Verification items for the finished model (mm, model axes). Face numbers are marked on the shaded views. Coordinates: 2 decimals unless noted, no trailing zeros. Order: outer loops, then holes, each group sorted by start corner. A loop starts at its lowest first (then second) coordinate and runs counter-clockwise, first axis right, second up. Notation, with made-up numbers: M -32.5,32.25 L 17.5,32.25 A31 ccw 17.5,64.25 Z; hole C 58.25,20.5 d4. An arc over 180 degrees is marked long. Write item = value, one per line.
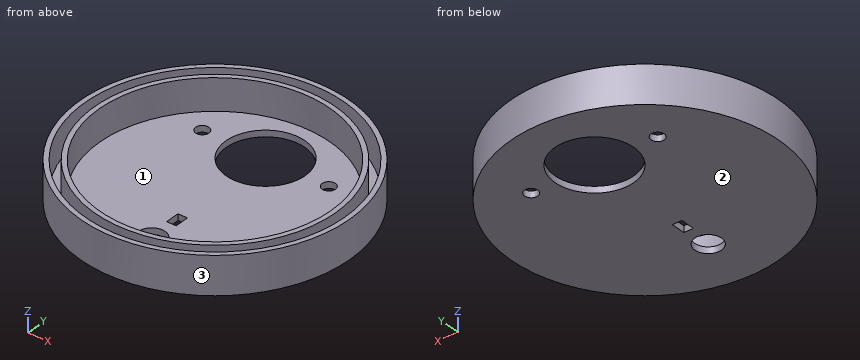
Autodesk Inventor part; units mm, degrees
sketch "Sketch1" plane through (0, 0, 0) normal (0, 0, 1) x (1, 0, 0)
  line L0 (0, 2.8582) -> (0, -2.8582) construction
  line L1 (-5.7775, 0) -> (5.7775, 0) construction
  circle A0 centre (0, 0) radius 42.5
  dimension "d0" = 85
extrude "Extrusion1" add sketch "Sketch1" along normal blind 2
sketch "Sketch2" plane through (0, 0, 2) normal (0, 0, 1) x (1, 0, 0)
  circle A0 centre (0, 0) radius 41
  circle A1 centre (0, 0) radius 38
  circle A2 centre (0, 0) radius 42.5
  circle A3 centre (0, 0) radius 36.5
  dimension "d3" = 82
  dimension "d4" = 76
  dimension "d5" = 73
extrude "Extrusion2" add sketch "Sketch2" along normal blind 10
sketch "Sketch3" plane through (0, 0, 0) normal (0, 0, -1) x (-1, 0, 0)
  circle A0 centre (0, 0) radius 42.5
  circle A1 centre (0, -25) radius 4.25
  line L0 (-59.5, 0) -> (59.5, 0)
  line L1 (1.5, -17.25) -> (-1.5, -17.25)
  line L2 (-1.5, -17.25) -> (-1.5, -12.75)
  line L3 (-1.5, -12.75) -> (1.5, -12.75)
  line L4 (1.5, -12.75) -> (1.5, -17.25)
  line L5 (1.5, -17.25) -> (-1.5, -12.75) construction
  line L6 (-1.5, -17.25) -> (1.5, -12.75) construction
  line L7 (0, -59.5) -> (0, 59.5)
  circle A2 centre (0, 20) radius 12.5
  point P0 (0, -15)
  dimension "d8" = 8.5
  dimension "d9" = 25
  dimension "d11" = 3
  dimension "d12" = 4.5
  dimension "d13" = 15
  dimension "d14" = 25
  dimension "d15" = 20
extrude "Extrusion3" cut sketch "Sketch3" against normal up to surface (2 mm away) contours A2 L7 | L7 A2 | L7 A1 | A1 L7 | L7 L1 L2 L3 | L3 L4 L1 L7
sketch "Sketch4" plane through (0, 0, 0) normal (0, 0, -1) x (-1, 0, 0)
  circle A0 centre (0, -25) radius 4.25
  circle A1 centre (0, 20) radius 12.5
  line L0 (1.5, -12.75) -> (-1.5, -12.75)
  line L1 (-1.5, -12.75) -> (-1.5, -17.25)
  line L2 (-1.5, -17.25) -> (1.5, -17.25)
  line L3 (1.5, -17.25) -> (1.5, -12.75)
  circle A2 centre (0, 0) radius 42.5
  line L4 (-59.5, 0) -> (59.5, 0)
  point P0 (-20, 20)
  point P1 (20, 20)
  dimension "d18" = 20
  dimension "d19" = 20
  dimension "d20" = 20
  dimension "d21" = 20
hole "Hole1" at (20, 20, 0) at (-20, 20, 0) direction (0, 0, 1) diameter 4.2 end through all
properties part number "Reservoir Adapter" material "S235"
Item 1: Sectioned sample at D-D, the plane x = 20. Enter the section's corners in (y, z).
Report:
outline = M -37.5,0 L 17.9,0 L 17.9,2 L -30.53,2 L -30.53,12 L -32.31,12 L -32.31,2 L -35.79,2 L -35.79,12 L -37.5,12 Z; M 22.1,0 L 37.5,0 L 37.5,12 L 35.79,12 L 35.79,2 L 32.31,2 L 32.31,12 L 30.53,12 L 30.53,2 L 22.1,2 Z
Item 2: Release check for a two-part mould opening along X. For the marked faces 1, 2 and 3 record: pulls with the +X half, pulls with the -X half, needs draft (parallel to the pull), parting line crosses it, or undercut.
Report:
face_1 = undercut
face_2 = needs draft
face_3 = parting line crosses it
Item 3: Sectioned sample at A-A, the plane x = 0. Enter the section's corners in (y, z).
Report:
outline = M -42.5,0 L -29.25,0 L -29.25,2 L -36.5,2 L -36.5,12 L -38,12 L -38,2 L -41,2 L -41,12 L -42.5,12 Z; M -20.75,0 L -17.25,0 L -17.25,2 L -20.75,2 Z; M -12.75,0 L 7.5,0 L 7.5,2 L -12.75,2 Z; M 32.5,0 L 42.5,0 L 42.5,12 L 41,12 L 41,2 L 38,2 L 38,12 L 36.5,12 L 36.5,2 L 32.5,2 Z
Item 4: Gauge pin test, flat ends, axial feed: pin 1 (1 mm diameter, centred on y = 26, z = 4.5, fed in from -X); pin 2 (2 mm diameter, centred on x = -0.5, z = 1.5, fed in from -Y); pin 3 (2 mm diameter, centred on x = 21, y = 5.5, fed in from +Z); pin 4 (4 mm diameter, centred on x = 20, y = 20, fed in from +Z). Record the tip position at first contact, or that the pin passes through.
Report:
pin_1 = -34
pin_2 = -42.5
pin_3 = 2
pin_4 = through
Item 5: Scan lines: L1, parallel to Y at x = 0, z = 0.6; L2, parallel to Y at x = 0, z = 5; L3, parallel to X at y = 6, z = 7.75. Record each from-to range of solid material in increasing order. Write a range as from..to.
Report:
L1 = -42.5..-29.25, -20.75..-17.25, -12.75..7.5, 32.5..42.5
L2 = -42.5..-41, -38..-36.5, 36.5..38, 41..42.5
L3 = -42.07..-40.56, -37.52..-36, 36..37.52, 40.56..42.07
Item 6: Sectioned sample at B-B, the plane z = 4. Enter the section's corners in (x, y), then the cut area to 3 significant figures.
Report:
outline = C 0,0 d85; C 0,0 d76; hole C 0,0 d82; hole C 0,0 d73
area = 745 mm^2
Item 7: Sectioned sample at C-C, the plane y = -25. Enter the section's corners in (x, z), then the cut area to 3 significant figures.
Report:
outline = M -34.37,0 L -4.25,0 L -4.25,2 L -26.59,2 L -26.59,12 L -28.62,12 L -28.62,2 L -32.5,2 L -32.5,12 L -34.37,12 Z; M 4.25,0 L 34.37,0 L 34.37,12 L 32.5,12 L 32.5,2 L 28.62,2 L 28.62,12 L 26.59,12 L 26.59,2 L 4.25,2 Z
area = 198 mm^2
